from build123d import *

# Parameters (mm, degrees)
SKETCH1_W           = 254
SKETCH1_H           = 76.2
SKETCH1_R           = 3.429
BOSS_EXTRUDE1_DEPTH = 3.175
FILLET1_R           = 3.175
CUT_EXTRUDE1_DEPTH  = 133.629900946
FILLET3_R           = 3.175


with BuildPart() as part:
    # Sketch1 → Boss-Extrude1 (new body)
    with BuildSketch(Plane(origin=(0, 0, 0), x_dir=(1, 0, 0), z_dir=(0, 1, 0))):
        Rectangle(SKETCH1_W, SKETCH1_H)
        with Locations(Location((-114.3, 28.575, 0), (0, 0, 270))):
            Circle(SKETCH1_R, mode=Mode.SUBTRACT)
        with Locations(Location((-114.3, -28.575, 0), (0, 0, 270))):
            Circle(SKETCH1_R, mode=Mode.SUBTRACT)
        with Locations(Location((114.3, 27.94, 0), (0, 0, 270))):
            Circle(SKETCH1_R, mode=Mode.SUBTRACT)
        with Locations(Location((114.3, -27.94, 0), (0, 0, 270))):
            Circle(SKETCH1_R, mode=Mode.SUBTRACT)
    extrude(amount=BOSS_EXTRUDE1_DEPTH)

    # Fillet1
    fillet1_edges = [part.edges().sort_by_distance(p)[0] for p in [
        (127, 1.5875, 38.1),
        (-127, 1.5875, 38.1),
        (-127, 1.5875, -38.1),
        (127, 1.5875, -38.1),
    ]]
    fillet(fillet1_edges, radius=FILLET1_R)

    # Sketch2 → Cut-Extrude1 (cut, through all)
    with BuildSketch(Plane(origin=(0, 3.175, 0), x_dir=(1, 0, 0), z_dir=(0, 1, 0))):
        with BuildLine():
            ThreePointArc((-100.658473406, 19.969571877), (-101.112278779, 19.289061706), (-101.6, 18.632432877))
            Line((-101.6, 18.632432877), (-101.6, -18.632432877))
            ThreePointArc((-101.6, -18.632432877), (-101.112278779, -19.289061706), (-100.658473406, -19.969571877))
            Line((-100.658473406, -19.969571877), (-19.882677051, 0))
            Line((-19.882677051, 0), (-100.658473406, 19.969571877))
        make_face()
        Polygon((82.858895983, 25.4), (-80.290356657, 25.4), (1.284269663, 5.232939604), align=None)
        Polygon((82.858895983, -25.4), (1.284269663, -5.232939604), (-80.290356657, -25.4), align=None)
        with BuildLine():
            Line((100.658473406, 19.334571877), (22.451216377, 0))
            Line((22.451216377, 0), (100.658473406, -19.334571877))
            ThreePointArc((100.658473406, -19.334571877), (101.112278779, -18.654061706), (101.6, -17.997432877))
            Line((101.6, -17.997432877), (101.6, 17.997432877))
            ThreePointArc((101.6, 17.997432877), (101.112278779, 18.654061706), (100.658473406, 19.334571877))
        make_face()
    extrude(amount=-CUT_EXTRUDE1_DEPTH, mode=Mode.SUBTRACT)

    # Fillet3
    # the kernel refuses this fillet: 3.175 mm, written as the material it adds along each edge
    with BuildSketch(Plane(origin=(100.658473406, 3.175, 19.334571877), x_dir=(-0.9707736729696135, 0, -0.23999682470625738), z_dir=(0, -1, 0)), Plane(origin=(-100.658473406, 3.175, -19.969571877), x_dir=(0.9707736729696127, 0, 0.23999682470626046), z_dir=(0, -1, 0))) as fillet3_piece_1:
        with BuildLine():
            CenterArc((2.141800615, 3.175), FILLET3_R, 205.317347828, 64.682652172)
            ThreePointArc((-0.728250522, 1.817269737), (-0.336527011, 0.919694558), (0, 0))
            Line((0, 0), (2.141800615, 0))
        make_face()
    extrude(amount=3.175)
    with BuildSketch(Plane(origin=(22.451216377, 3.175, 0), x_dir=(0.9707736729695857, 0, -0.23999682470636963), z_dir=(0, -1, 0)), Plane(origin=(-19.882677051, 3.175, 0), x_dir=(-0.9707736729695856, 0, 0.23999682470636988), z_dir=(0, -1, 0))) as fillet3_piece_2:
        with BuildLine():
            CenterArc((FILLET3_R * 4.04494382022, FILLET3_R), FILLET3_R, 117.772705909, 152.227294091)
            Line((FILLET3_R * 3.57897862218, FILLET3_R * 1.88480304826), (0, 0))
            Line((0, 0), (FILLET3_R * 4.04494382022, 0))
        make_face()
    extrude(amount=3.175)
    with BuildSketch(Plane(origin=(100.658473406, 3.175, -19.334571877), x_dir=(-0.970773672969613, 0, 0.23999682470625897), z_dir=(0, -1, 0))) as fillet3_piece_3:
        with BuildLine():
            CenterArc((2.141800615, -3.175), FILLET3_R, 90, 64.682652172)
            ThreePointArc((-0.728250522, -1.817269737), (-0.336527011, -0.919694558), (0, 0))
            Line((0, 0), (2.141800615, 0))
        make_face()
    extrude(amount=3.175)
    with BuildSketch(Plane(origin=(82.858895983, 3.175, -25.4), x_dir=(-0.9707736729695856, 0, 0.23999682470636996), z_dir=(0, -1, 0)), Plane(origin=(-80.290356657, 3.175, 25.4), x_dir=(0.9707736729695856, 0, -0.23999682470636974), z_dir=(0, -1, 0)), Plane(origin=(-80.290356657, 3.175, -25.4), x_dir=(1, 0, 0), z_dir=(0, -1, 0))) as fillet3_piece_4:
        with BuildLine():
            CenterArc((FILLET3_R * 8.21166561425, FILLET3_R), FILLET3_R, 103.886352954, 166.113647046)
            Line((FILLET3_R * 7.97166878954, FILLET3_R * 1.97077367297), (0, 0))
            Line((0, 0), (FILLET3_R * 8.21166561425, 0))
        make_face()
    extrude(amount=3.175)
    with BuildSketch(Plane(origin=(82.858895983, 3.175, 25.4), x_dir=(-0.9707736729695857, 0, -0.2399968247063698), z_dir=(0, -1, 0))) as fillet3_piece_5:
        with BuildLine():
            CenterArc((FILLET3_R * 8.21166561425, -FILLET3_R), FILLET3_R, 90, 166.113647046)
            Line((FILLET3_R * 7.97166878954, -FILLET3_R * 1.97077367297), (0, 0))
            Line((0, 0), (FILLET3_R * 8.21166561425, 0))
        make_face()
    extrude(amount=3.175)
    with BuildSketch(Plane(origin=(-100.658473406, 3.175, 19.969571877), x_dir=(-0.5838848021252715, 0, -0.811836521626819), z_dir=(0, -1, 0))) as fillet3_piece_6:
        with BuildLine():
            CenterArc((2.150451203, 3.169147283), FILLET3_R, 201.837892452, 64.682652172)
            Line((-0.796710862, 1.988105047), (0, 0))
            ThreePointArc((0, 0), (0.978879221, 0.029731803), (1.957758443, 0))
        make_face()
    extrude(amount=3.175)
    with BuildSketch(Plane(origin=(1.284269663, 3.175, -5.232939604), x_dir=(0.9707736729695848, 0, -0.23999682470637296), z_dir=(0, -1, 0))) as fillet3_piece_7:
        with BuildLine():
            CenterArc((FILLET3_R * 0.247222222222, -FILLET3_R), FILLET3_R, 90, 27.772705909)
            Line((-FILLET3_R * 0.21874297582, -FILLET3_R * 0.115196951738), (0, 0))
            Line((0, 0), (FILLET3_R * 0.247222222222, 0))
        make_face()
    extrude(amount=3.175)
    with BuildSketch(Plane(origin=(1.284269663, 3.175, 5.232939604), x_dir=(0.9707736729695816, 0, 0.23999682470638586), z_dir=(0, -1, 0))) as fillet3_piece_8:
        with BuildLine():
            CenterArc((FILLET3_R * 0.247222222222, FILLET3_R), FILLET3_R, 242.227294091, 27.772705909)
            Line((-FILLET3_R * 0.21874297582, FILLET3_R * 0.115196951738), (0, 0))
            Line((0, 0), (FILLET3_R * 0.247222222222, 0))
        make_face()
    extrude(amount=3.175)
    with BuildSketch(Plane(origin=(101.6, 3.175, -17.997432877), x_dir=(0, 0, 1), z_dir=(0, -1, 0)), Plane(origin=(-101.6, 3.175, 18.632432877), x_dir=(0, 0, -1), z_dir=(0, -1, 0))) as fillet3_piece_9:
        with BuildLine():
            CenterArc((1.040546779, 3.175), FILLET3_R, 235.322589412, 34.677410588)
            ThreePointArc((-0.765886428, 0.563980263), (-0.378785041, 0.28763694), (0, 0))
            Line((0, 0), (1.040546779, 0))
        make_face()
    extrude(amount=3.175)
    with BuildSketch(Plane(origin=(101.6, 3.175, 17.997432877), x_dir=(-0.5929556750159476, 0, 0.8052351007416294), z_dir=(0, -1, 0))) as fillet3_piece_10:
        with BuildLine():
            CenterArc((1.044749477, 3.173619563), FILLET3_R, 233.63296639, 34.677410588)
            Line((-0.837884791, 0.616998118), (0, 0))
            ThreePointArc((0, 0), (0.475566966, 0.007012621), (0.951133933, 0))
        make_face()
    extrude(amount=3.175)
    with BuildSketch(Plane(origin=(-101.6, 3.175, -18.632432877), x_dir=(0, 0, 1), z_dir=(0, -1, 0))) as fillet3_piece_11:
        with BuildLine():
            CenterArc((1.040546779, -3.175), FILLET3_R, 90, 34.677410588)
            ThreePointArc((-0.765886428, -0.563980263), (-0.378785041, -0.28763694), (0, 0))
            Line((0, 0), (1.040546779, 0))
        make_face()
    extrude(amount=3.175)


solid = part.part
Check sheet for the modelled part. Datum: model origin and axes. Units: mm. A direction names the side the tool comes from. Coordinates: 2 decimals unless noted, no trailing zeros. Write each loop counter-clockwise with the first axis right and the second up, starting at its lowest first coordinate (ties: lowest second). Pieces come first, ordered by that corner, then holes.
Item 1: Cross-section at A-A on x = -114.3. Record the boundary of the cut face in (y, z) (3 decimals), then the cut area to 3 significant figures.
Numbers:
outline: (0, -38.1) - (3.175, -38.1) - (3.175, -32.004) - (0, -32.004) - close; (0, -25.146) - (3.175, -25.146) - (3.175, 25.146) - (0, 25.146) - close; (0, 32.004) - (3.175, 32.004) - (3.175, 38.1) - (0, 38.1) - close
area: 198 mm2
Item 2: Depth check by flat-ended pin: pin 1 Ø11 at (x, z) = (-114.3, 28.575) entering from +Y (3 decimals). Enter the tip coordinate at first touch or a pass-through.
Numbers:
pin 1: stops at y = 3.175
Item 3: Scan lines: probe 1 along Z at (x, y) = (112.5, 2.5); probe 2 along X at (y, z) = (0.85, 27.94); probe 3 along X at (y, z) = (2.15, -1). Record each from-to range of solid material in increasing order.
Numbers:
probe 1: z = -38.1 to -30.86, -25.02 to 25.02, 30.86 to 38.1
probe 2: x = -127 to -117.67, -110.93 to 110.87, 117.73 to 127
probe 3: x = -127 to -101.6, -30.1 to 32.67, 101.6 to 127
Item 4: Mould release check, pull along Z, two halves, no side actions. Record for faces 3 (the face through (30.19, 1.61, 12.38)), 4 (the face through (-2, 0, 1)): released by +Z, released by -Z, zero draft, split by the parting line, or undercut.
Numbers:
face 3: undercut
face 4: zero draft
Item 5: Cross-section at D-D on y = 2.6. Count the separate pieces of the cut face and the enclosed holes in it, then the cut area to 3 significant figures.
Numbers:
separate pieces: 1
enclosed holes: 8
area: 13,000 mm2
Item 6: Cross-section at C-C on x = -77.5. Record the boundary of the cut face in (y, z) (3 decimals), then the cut area to 3 significant figures.
Numbers:
outline: (0, -38.1) - (3.175, -38.1) - (3.175, -14.244) - (0, -14.244) - close; (0, 14.244) - (3.175, 14.244) - (3.175, 38.1) - (0, 38.1) - close
area: 151 mm2
Item 7: Cross-section at B-B on z = 27.94. Record the boundary of the cut face in (x, y) (3 decimals), then the cut area to 3 significant figures.
Numbers:
outline: (-127, 0) - (-117.67, 0) - (-117.67, 3.175) - (-127, 3.175) - close; (-110.93, 0) - (110.871, 0) - (110.871, 3.175) - (-110.93, 3.175) - close; (117.729, 0) - (127, 0) - (127, 3.175) - (117.729, 3.175) - close
area: 763 mm2
Item 8: Access from +Z, -Z, +X, -X, +Y, -Y to the whole of each face (thin tool, end or side, straight path). Record for faces 1 (the face through (-2, 3.175, 1)), 2 (the face through (67.19, 1.61, -11.06)).
Numbers:
face 1: +Z, -Z, +X, -X, +Y
face 2: +Y, -Y
